```python
from build123d import *

# Parameters (mm, degrees)
SKETCH1_R           = 2.54
BOSS_EXTRUDE1_DEPTH = 3.048


with BuildPart() as part:
    # Sketch1 → Boss-Extrude1 (new body)
    with BuildSketch(Plane(origin=(0, 0, 0), x_dir=(1, 0, 0), z_dir=(0, 1, 0))):
        Polygon((0, 20.32), (0, 0), (-6.35, 0), (-6.35, -33.02), (16.51, -33.02), (49.550989027, 5.566695169), (100.350989027, 5.566695169), (100.350989027, 23.346695169), (13.97, 53.34), (-6.35, 53.34), (-6.35, 20.32), align=None)
        with Locations((8.255, 10.16)):
            Circle(SKETCH1_R, mode=Mode.SUBTRACT)
        with Locations((87.689183737, 15.726695169)):
            Circle(SKETCH1_R, mode=Mode.SUBTRACT)
        with Locations((6.35, -24.13)):
            Circle(SKETCH1_R, mode=Mode.SUBTRACT)
        with Locations((6.35, 44.45)):
            Circle(SKETCH1_R, mode=Mode.SUBTRACT)
        with Locations((67.330989027, 15.726695169)):
            Circle(SKETCH1_R, mode=Mode.SUBTRACT)
    extrude(amount=BOSS_EXTRUDE1_DEPTH)


solid = part.part
```
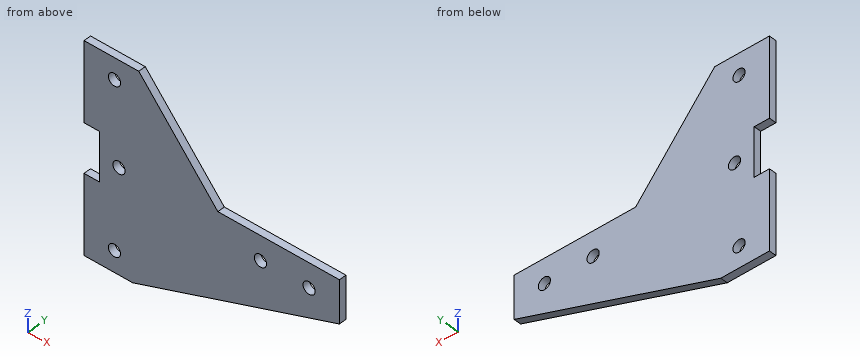
Read the model definition and answer for the solid it produces. Units are mm, in the model's axes. Give positions to 0.01 mm unless a question says otherwise; leave off trailing zeros. Order: outer loops, then holes, each group sorted by start corner. A loop starts at its lowest first (then second) coordinate and runs counter-clockwise, first axis right, second up. Notation, with made-up numbers: (57, -40) -> (95, -40) arc R12 cw to (95, -20) -> close; hole circle Ø3 at (77, 42.25). An arc over 180 degrees is marked (long way). Write item = value, one per line.
1. A cutting plane is placed at D-D, the plane x = 63. Write down the section's boundary in (y, z).
Numbers:
outline = (0, -36.32) -> (3.05, -36.32) -> (3.05, -5.57) -> (0, -5.57) -> close
2. Straight lines are drawn through the part: line 1 along Z through (x, y) = (6.35, 1.2); line 2 along X through (y, z) = (1.5, -10.16) (3 decimals); line 3 along Z through (x, y) = (9, 0.2). For each, find the intervals that lie inside material, in ascending order.
Numbers:
line_1 = -53.34 to -46.99, -41.91 to -11.84, -8.48 to 21.59, 26.67 to 33.02
line_2 = 0 to 5.715, 10.795 to 100.351
line_3 = -53.34 to -12.59, -7.73 to 33.02
3. A cutting plane is placed at B-B, the plane y = 0.9. Write down the section's boundary in (x, z) (3 decimals), and give its area (3 significant figures).
Numbers:
outline = (-6.35, -53.34) -> (13.97, -53.34) -> (100.351, -23.347) -> (100.351, -5.567) -> (49.551, -5.567) -> (16.51, 33.02) -> (-6.35, 33.02) -> (-6.35, 0) -> (0, 0) -> (0, -20.32) -> (-6.35, -20.32) -> close; hole circle Ø5.08 at (6.35, -44.45); hole circle Ø5.08 at (6.35, 24.13); hole circle Ø5.08 at (8.255, -10.16); hole circle Ø5.08 at (67.331, -15.727); hole circle Ø5.08 at (87.689, -15.727)
area = 5,090 mm²
4. A cutting plane is placed at A-A, the plane z = -10.16. Write down the section's boundary in (x, y) (3 decimals).
Numbers:
outline = (0, 0) -> (5.715, 0) -> (5.715, 3.048) -> (0, 3.048) -> close; (10.795, 0) -> (100.351, 0) -> (100.351, 3.048) -> (10.795, 3.048) -> close
5. A cutting plane is placed at C-C, the plane z = 24.13. Write down the section's boundary in (x, y), and give its area (3 significant figures).
Numbers:
outline = (-6.35, 0) -> (3.81, 0) -> (3.81, 3.05) -> (-6.35, 3.05) -> close; (8.89, 0) -> (24.12, 0) -> (24.12, 3.05) -> (8.89, 3.05) -> close
area = 77.4 mm²
